Check sheet for the modelled part. Datum: model origin and axes. Units: mm. Face numbers are marked on the shaded views. A direction names the side the tool comes from. Give positions to 0.01 mm unless a question says otherwise; leave off trailing zeros. Write each loop counter-clockwise with the first axis right and the second up, starting at its lowest first coordinate (ties: lowest second). Pieces come first, ordered by that corner, then holes. Notation, with made-up numbers: (52, 42.5) -> (73, 42.5) arc R33 cw to (73, 74.5) -> close; hole circle Ø5 at (-26.5, 65). An arc over 180 degrees is marked (long way). Use a Markdown table: item, result. Add a question column.
1. Gauge pin test, flat ends, axial feed: P1, Ø13, axis at x = 25.5, y = 6.5, coming from the -Z side; P2, Ø3.5, axis at x = -27.5, y = -3.5, coming from the -Z side; P3, Ø1.9, axis at y = -6, z = -1.5, coming from the +X side. Record the tip position at first contact, or that the pin passes through.
2. Set-up check for the marked faces 5 and 6: record each of +Z, -Z, +X, -X, +Y, -Y from which the full face is reachable in a straight line by a thin tool's end or side.
3. Scan lines: probe 1 along Z at (x, y) = (-6.5, -9); probe 2 along X at (y, z) = (14, 1); probe 3 along X at (y, z) = (-6, -4.5). Record each from-to range of solid material in increasing order. Write a range as [from, to].
4. Cross-section at A-A (z = -5.5). Enter the section's corners in (x, y), then the cut area to 3 significant figures.
5. Release check for a two-part mould opening along X. For the marked faces 1, 2, 3 and 4 record: released by +X, released by -X, zero draft, split by the parting line, or undercut.
6. Cross-section at B-B (x = 29). Enter the section's corners in (y, z).
7. Cross-section at C-C (y = 2.5). Enter the section's corners in (x, z), then the cut area to 3 significant figures.
8. Cross-section at D-D (z = -2.25). Enter the section's corners in (x, y).
from build123d import *

# Parameters (mm, degrees)
SKETCH1_W            = 50
SKETCH1_H            = 32
BOSS_EXTRUDE1_DEPTH  = 3.75
BOSS_EXTRUDE2_DEPTH  = 32
SKETCH4_W            = 8
SKETCH4_H            = 3.75
BOSS_EXTRUDE3_DEPTH  = 32
M2_CLEARANCE_HOLE1_D = 2.4


with BuildPart() as part:
    # Sketch1 → Boss-Extrude1 (new body)
    with BuildSketch(Plane.XY):
        Rectangle(SKETCH1_W, SKETCH1_H)
    extrude(amount=BOSS_EXTRUDE1_DEPTH)

    # Sketch2 → Boss-Extrude2 (add)
    with BuildSketch(Plane(origin=(0, 16, 0), x_dir=(1, 0, 0), z_dir=(0, 1, 0))):
        Polygon((-21.25, 0), (-21.25, 6.363961031), (-14.886038969, 0), align=None)
        Polygon((14.886038969, 0), (21.25, 0), (21.25, 6.363961031), align=None)
    extrude(amount=-BOSS_EXTRUDE2_DEPTH)

    # Sketch4 → Boss-Extrude3 (add)
    with BuildSketch(Plane(origin=(0, 16, 0), x_dir=(1, 0, 0), z_dir=(0, 1, 0))):
        with Locations((29, -1.875)):
            Rectangle(SKETCH4_W, SKETCH4_H)
        with Locations((-29, -1.875)):
            Rectangle(SKETCH4_W, SKETCH4_H)
    extrude(amount=-BOSS_EXTRUDE3_DEPTH)

    # M2 Clearance Hole1 (through all)
    with Locations(Plane.XY.offset(3.75)):
        with Locations((-29.16173141, -12.975), (-29.16173141, 12.975)):
            m2_clearance_hole1 = Hole(M2_CLEARANCE_HOLE1_D / 2)

    # Mirror1: M2 Clearance Hole1 across plane
    add(m2_clearance_hole1.mirror(Plane(origin=(0, 0, 0), x_dir=(0, 0, 1), z_dir=(1, 0, 0))), mode=Mode.SUBTRACT)


solid = part.part
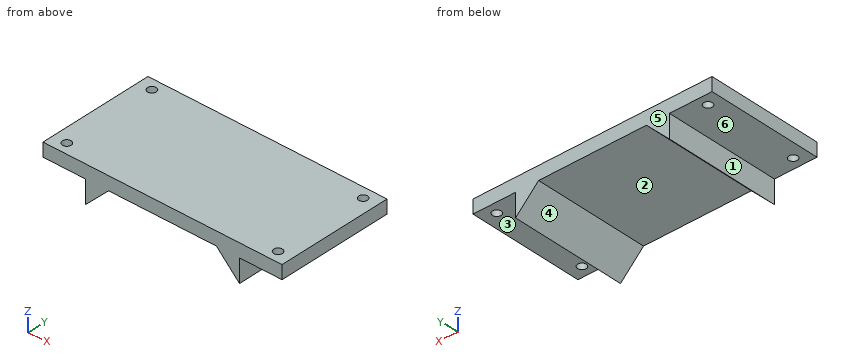
Worked answers:
| question | item | result |
|---|---|---|
| 1 | P1 | stops at z = -6.36 |
| 1 | P2 | stops at z = 0 |
| 1 | P3 | stops at x = 21.25 |
| 2 | face 5 | +Z, -Z, +X, -X, +Y |
| 2 | face 6 | -Z, -X, +Y, -Y |
| 3 | probe 1 | z = [0, 3.75] |
| 3 | probe 2 | x = [-33, -29.79], [-28.54, 28.54], [29.79, 33] |
| 3 | probe 3 | x = [-21.25, -19.39], [19.39, 21.25] |
| 4 | outline | (-21.25, -16) -> (-20.39, -16) -> (-20.39, 16) -> (-21.25, 16) -> close; (20.39, -16) -> (21.25, -16) -> (21.25, 16) -> (20.39, 16) -> close |
| 4 | area | 55.3 mm² |
| 5 | face 1 | released by -X |
| 5 | face 2 | undercut |
| 5 | face 3 | zero draft |
| 5 | face 4 | undercut |
| 6 | outline | (-16, 0) -> (-14.16, 0) -> (-14.16, 3.75) -> (-16, 3.75) -> close; (-11.79, 0) -> (11.79, 0) -> (11.79, 3.75) -> (-11.79, 3.75) -> close; (14.16, 0) -> (16, 0) -> (16, 3.75) -> (14.16, 3.75) -> close |
| 7 | outline | (-33, 0) -> (-21.25, 0) -> (-21.25, -6.36) -> (-14.89, 0) -> (14.89, 0) -> (21.25, -6.36) -> (21.25, 0) -> (33, 0) -> (33, 3.75) -> (-33, 3.75) -> close |
| 7 | area | 288 mm² |
| 8 | outline | (-21.25, -16) -> (-17.14, -16) -> (-17.14, 16) -> (-21.25, 16) -> close; (17.14, -16) -> (21.25, -16) -> (21.25, 16) -> (17.14, 16) -> close |
